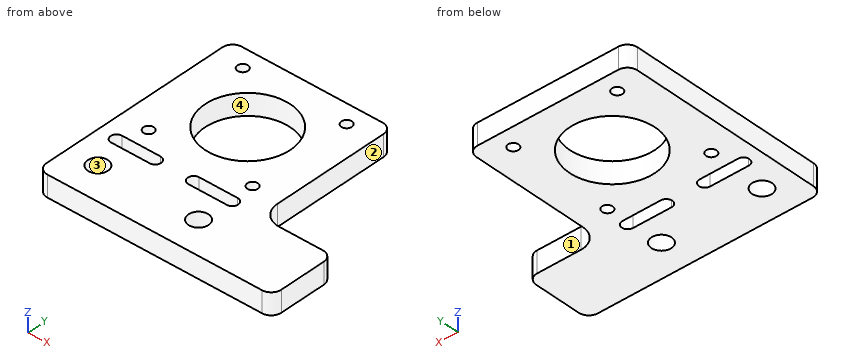
```python
from build123d import *

# Parameters (mm, degrees)
SKETCH1_R           = 2.9845
SKETCH1_R_2         = 1.562499999
SKETCH1_R_3         = 12.7
BOSS_EXTRUDE1_DEPTH = 6.35


with BuildPart() as part:
    # Sketch1 → Boss-Extrude1 (new body)
    with BuildSketch(Plane.XY):
        with BuildLine():
            Line((363.683701588, 169.033854224), (427.683701589, 169.033854224))
            ThreePointArc((427.683701589, 169.033854224), (429.805021933, 169.912533881), (430.68370159, 172.033854225))
            Line((430.68370159, 172.033854225), (430.68370159, 186.033854223))
            ThreePointArc((430.68370159, 186.033854223), (429.805021933, 188.155174567), (427.683701588, 189.033854223))
            Line((427.683701588, 189.033854223), (414.683701589, 189.033854223))
            ThreePointArc((414.683701589, 189.033854223), (410.4410609, 190.791213536), (408.683701587, 195.033854224))
            Line((408.683701587, 195.033854224), (408.683701587, 230.033854224))
            ThreePointArc((408.683701587, 230.033854224), (407.805021931, 232.155174567), (405.683701588, 233.033854223))
            Line((405.683701588, 233.033854223), (363.683701587, 233.033854223))
            ThreePointArc((363.683701587, 233.033854223), (361.562381244, 232.155174567), (360.683701588, 230.033854224))
            Line((360.683701588, 230.033854224), (360.683701588, 172.033854225))
            ThreePointArc((360.683701588, 172.033854225), (361.562381244, 169.912533881), (363.683701588, 169.033854224))
        make_face()
        with Locations((369.683701589, 179.033854223)):
            Circle(SKETCH1_R, mode=Mode.SUBTRACT)
        with Locations((399.683701589, 179.033854223)):
            Circle(SKETCH1_R, mode=Mode.SUBTRACT)
        with Locations((369.189701589, 196.313382783)):
            Circle(SKETCH1_R_2, mode=Mode.SUBTRACT)
        with Locations((400.177701589, 196.313382783)):
            Circle(SKETCH1_R_2, mode=Mode.SUBTRACT)
        with Locations((384.683701589, 211.807382783)):
            Circle(SKETCH1_R_3, mode=Mode.SUBTRACT)
        with Locations((369.189701589, 227.301382783)):
            Circle(SKETCH1_R_2, mode=Mode.SUBTRACT)
        with Locations((400.177701589, 227.301382783)):
            Circle(SKETCH1_R_2, mode=Mode.SUBTRACT)
        with BuildLine():
            Line((366.183701588, 187.299538128), (377.683701588, 187.299538128))
            ThreePointArc((377.683701588, 187.299538128), (379.433701588, 189.049538128), (377.683701588, 190.799538128))
            Line((377.683701588, 190.799538128), (366.183701588, 190.799538128))
            ThreePointArc((366.183701588, 190.799538128), (364.433701588, 189.049538128), (366.183701588, 187.299538128))
        make_face(mode=Mode.SUBTRACT)
        with BuildLine():
            Line((389.183701588, 187.299538128), (400.683701588, 187.299538128))
            ThreePointArc((400.683701588, 187.299538128), (402.433701588, 189.049538128), (400.683701588, 190.799538128))
            Line((400.683701588, 190.799538128), (389.183701588, 190.799538128))
            ThreePointArc((389.183701588, 190.799538128), (387.433701588, 189.049538128), (389.183701588, 187.299538128))
        make_face(mode=Mode.SUBTRACT)
    extrude(amount=BOSS_EXTRUDE1_DEPTH)


solid = part.part
```
Can you work these out from the model? Positions are in its coordinate system, mm. Face numbers are marked on the shaded views. Give positions to 0.01 mm unless a question says otherwise; leave off trailing zeros. Loops run counter-clockwise (first coordinate to the right, second up) from the corner with the lowest first, then second, coordinate; pieces in that order, holes last. Notation, with made-up numbers: M 38,-19.5 L 52,-19.5 A20 cw 52,-7.5 Z; hole C -16,-11.75 d3. An arc over 180 degrees is marked long. Use one line per item in the form item = value. Start each with the question number.
(1) I want a section at B-B, the plane y = 177. Write out the boundary of the cut face in (x, z).
(2) Please list where these lines run through material, in increasing order: line 1 (Y direction, x = 377.5, z = 3); line 2 (Y direction, x = 375.5, z = 4.5); line 3 (X direction, y = 226, z = 4).
(3) I'm going to push flat-ended pins straight in: P1, Ø1.9, axis at x = 369.19, y = 196.31, coming from the +Z side; P2, Ø3, axis at x = 372.5, y = 191, coming from the -Z side; P3, Ø1.9, axis at x = 419.5, z = 3, coming from the +Y side. Where does each tip first touch, or does it pass through?
(4) I want a section at A-A, the plane x = 375.5. Write out the boundary of the cut face in (y, z).
(5) Thinking about a two-plate mould opening in X: for the marked faces 1, 2, 3 and 4, which applies, released by +X, released by -X, zero draft, split by the parting line, or undercut?
(6) I want a section at D-D, the plane y = 223.5. Write out the boundary of the cut face in (x, z), and give its area (3 significant figures).
(7) I want a section at C-C, the plane z = 1.75. State how many separate pieces and enclosed holes the cut face has, and give its area (3 significant figures).
Worked out:
q1.outline = M 360.68,0 L 367.5,0 L 367.5,6.35 L 360.68,6.35 Z; M 371.87,0 L 397.5,0 L 397.5,6.35 L 371.87,6.35 Z; M 401.87,0 L 430.68,0 L 430.68,6.35 L 401.87,6.35 Z
q2.line_1 = 169.03 to 187.3, 190.8 to 201.33, 222.28 to 233.03
q2.line_2 = 169.03 to 187.3, 190.8 to 203.04, 220.58 to 233.03
q2.line_3 = 360.68 to 368.32, 370.05 to 399.31, 401.04 to 408.68
q3.P1 = through
q3.P2 = 0
q3.P3 = 189.03
q4.outline = M 169.03,0 L 187.3,0 L 187.3,6.35 L 169.03,6.35 Z; M 190.8,0 L 203.04,0 L 203.04,6.35 L 190.8,6.35 Z; M 220.58,0 L 233.03,0 L 233.03,6.35 L 220.58,6.35 Z
q5.face_1 = zero draft
q5.face_2 = released by +X
q5.face_3 = undercut
q5.face_4 = undercut
q6.outline = M 360.68,0 L 379.73,0 L 379.73,6.35 L 360.68,6.35 Z; M 389.64,0 L 408.68,0 L 408.68,6.35 L 389.64,6.35 Z
q6.area = 242 mm²
q7.separate_pieces = 1
q7.enclosed_holes = 9
q7.area = 2,820 mm²
